Check sheet for the modelled part. Datum: model origin and axes. Units: mm. Face numbers are marked on the shaded views. A direction names the side the tool comes from. Coordinates: 2 decimals unless noted, no trailing zeros. Order: outer loops, then holes, each group sorted by start corner. A loop starts at its lowest first (then second) coordinate and runs counter-clockwise, first axis right, second up.
1. Thickness scan on line 1 (Z direction, x = -25.5, y = -32.5); line 2 (Y direction, x = 0, z = 78); line 3 (Y direction, x = 0, z = 219). Record the ranges inside material, lowest first.
2. Cross-section at C-C (y = 28.5). Enter the section's corners in (x, z), then the cut area to 3 significant figures.
3. Gauge pin test, flat ends, axial feed: pin 1 Ø1.5 at (x, z) = (-7.5, 205) entering from +Y; pin 2 Ø1 at (y, z) = (-26, 55) entering from +X; pin 3 Ø1.5 at (y, z) = (27.5, 75) entering from +X. Record the tip position at first contact, or that the pin passes through.
4. Cross-section at A-A (y = 0). Enter the section's corners in (x, z), then the cut area to 3 significant figures.
5. Set-up check for the marked faces 1 and 2: record each of +Z, -Z, +X, -X, +Y, -Y from which the full face is reachable in a straight line by a thin tool's end or side.
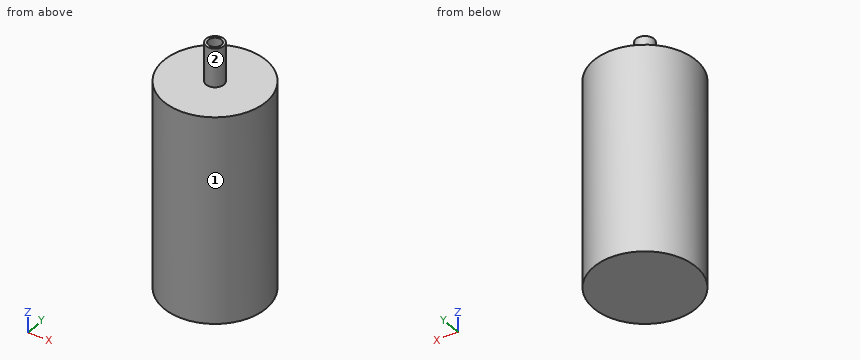
```python
from build123d import *

# Parameters (mm, degrees)
F0_R     = 50
F0_R_2   = 49
F1_DEPTH = 201
F2_R     = 50
F3_DEPTH = 1
F5_R     = 50
F5_R_2   = 6.35
F6_DEPTH = 1
F8_R     = 8.73125
F8_R_2   = 6.35
F9_DEPTH = 38


with BuildPart() as f1:
    # F0 (on Top) → F1 (new body)
    with BuildSketch(Plane.XY):
        Circle(F0_R)
        Circle(F0_R_2, mode=Mode.SUBTRACT)
    extrude(amount=F1_DEPTH)

    # F2 (on face) → F3 (join)
    with BuildSketch(Plane(origin=(0, 0, 0), x_dir=(1, 0, 0), z_dir=(0, 0, -1))):
        Circle(F2_R)
    extrude(amount=F3_DEPTH)

    # F5 (on offset) → F6 (join)
    with BuildSketch(Plane.XY.offset(201)):
        Circle(F5_R)
        Circle(F5_R_2, mode=Mode.SUBTRACT)
    extrude(amount=F6_DEPTH)

    # F8 (on offset) → F9 (join)
    with BuildSketch(Plane.XY.offset(202)):
        Circle(F8_R)
        Circle(F8_R_2, mode=Mode.SUBTRACT)
    extrude(amount=F9_DEPTH)


solid = f1.part
```
Data:
1. line 1: z = -1 to 0, 201 to 202
1. line 2: y = -50 to -49, 49 to 50
1. line 3: y = -8.73 to -6.35, 6.35 to 8.73
2. outline: (-41.08, -1) - (41.08, -1) - (41.08, 202) - (-41.08, 202) - close; hole (-39.86, 0) - (39.86, 0) - (39.86, 201) - (-39.86, 201) - close
2. area: 656 mm2
3. pin 1: stops at y = 5.54
3. pin 2: stops at x = 43.01
3. pin 3: stops at x = 42.24
4. outline: (-50, -1) - (50, -1) - (50, 202) - (8.73, 202) - (8.73, 240) - (6.35, 240) - (6.35, 201) - (49, 201) - (49, 0) - (-49, 0) - (-49, 201) - (-6.35, 201) - (-6.35, 240) - (-8.73, 240) - (-8.73, 202) - (-50, 202) - close
4. area: 770 mm2
5. face 1: +Z, -Z
5. face 2: +Z
